Geometry check sheet. Reference: the model listing, model coordinates, mm. Round coordinates to 2 decimals unless told otherwise and drop trailing zeros. Loops run counter-clockwise (first coordinate to the right, second up) from the corner with the lowest first, then second, coordinate; pieces in that order, holes last.
```python
from build123d import *

# Parameters (mm, degrees)
SKETCH_1_R      = 2
SKETCH_1_R_2    = 1.99
EXTRUDE_1_DEPTH = 3


with BuildPart() as part:
    # 草图1 → 凸台-拉伸1 (new body)
    with BuildSketch(Plane.XY):
        with BuildLine():
            Line((-16.651457747, -45.984160086), (-16.651457747, -35.65505653))
            Line((-16.651457747, -35.65505653), (-36.651457747, -35.65505653))
            Line((-36.651457747, -35.65505653), (-36.651457747, -75.65505653))
            Line((-36.651457747, -75.65505653), (14.818542253, -75.65505653))
            Line((14.818542253, -75.65505653), (39.818542253, -32.353786341))
            Line((39.818542253, -32.353786341), (22.498034177, -22.353786341))
            ThreePointArc((22.498034177, -22.353786341), (8.713172451, -39.144030649), (-9.741633911, -50.605044516))
            ThreePointArc((-9.741633911, -50.605044516), (-14.430925396, -50.140427593), (-16.651457747, -45.984160086))
        make_face()
        with Locations((-26.651457747, -40.65505653)):
            Circle(SKETCH_1_R, mode=Mode.SUBTRACT)
        with Locations((-26.651457747, -50.65505653)):
            Circle(SKETCH_1_R_2, mode=Mode.SUBTRACT)
        with Locations((-20.181457747, -65.65505653)):
            Circle(SKETCH_1_R, mode=Mode.SUBTRACT)
        with Locations((-5.181457747, -65.65505653)):
            Circle(SKETCH_1_R, mode=Mode.SUBTRACT)
        with Locations((16.158288215, -53.334548455)):
            Circle(SKETCH_1_R, mode=Mode.SUBTRACT)
        with Locations((23.658288215, -40.344167398)):
            Circle(SKETCH_1_R, mode=Mode.SUBTRACT)
    extrude(amount=EXTRUDE_1_DEPTH)


solid = part.part
```
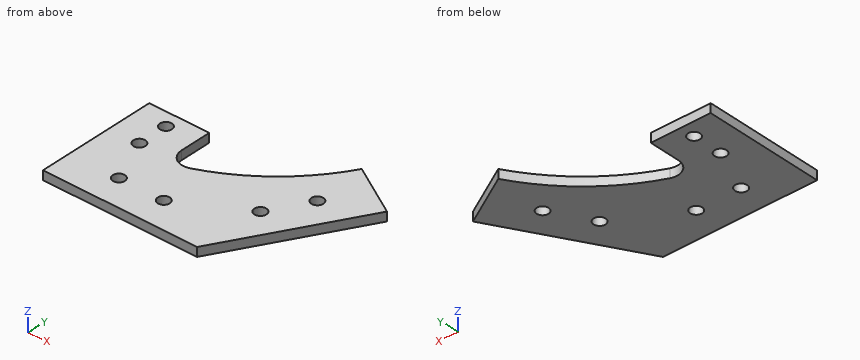
1) Scan lines: line 1 along X through (y, z) = (-41, 0.3); line 2 along Y through (x, z) = (-27.5, 1.05); line 3 along X through (y, z) = (-55, 0.25). Record each from-to range of solid material in increasing order.
Report:
line 1: x = -36.65 to -28.62, -24.68 to -16.65, 6.5 to 21.77, 25.55 to 34.83
line 2: y = -75.66 to -52.46, -48.86 to -42.47, -38.84 to -35.66
line 3: x = -36.65 to 15.05, 17.27 to 26.74
2) Sectioned sample at B-B, the plane y = -47. Record the cut outline in (x, z), then the cut area to 3 significant figures.
Report:
outline: (-36.65, 0) - (-16.55, 0) - (-16.55, 3) - (-36.65, 3) - close; (-2.35, 0) - (31.36, 0) - (31.36, 3) - (-2.35, 3) - close
area: 161 mm2
3) Sectioned sample at C-C, the plane x = -10.5. Record the cut outline in (y, z), then the cut area to 3 significant figures.
Report:
outline: (-75.66, 0) - (-50.85, 0) - (-50.85, 3) - (-75.66, 3) - close
area: 74.4 mm2
4) Sectioned sample at D-D, the plane y = -37. Record the cut outline in (x, z).
Report:
outline: (-36.65, 0) - (-16.65, 0) - (-16.65, 3) - (-36.65, 3) - close; (11.05, 0) - (37.14, 0) - (37.14, 3) - (11.05, 3) - close
5) Gauge pin test, flat ends, axial feed: pin 1 (1 mm diameter, centred on x = 18.5, z = 1, fed in from +Y); pin 2 (5 mm diameter, centred on x = -5.18, y = -65.66, fed in from -Z); pin 3 (3 mm diameter, centred on x = -26.65, y = -50.66, fed in from -Z). Record the tip position at first contact, or that the pin passes through.
Report:
pin 1: stops at y = -27.79
pin 2: stops at z = 0
pin 3: passes through
6) Sectioned sample at A-A, the plane z = 0.85. Record the cut outline in (x, y).
Report:
outline: (-36.65, -75.66) - (14.82, -75.66) - (39.82, -32.35) - (22.5, -22.35) arc R66.6 cw to (-9.74, -50.61) arc R5 cw to (-16.65, -45.98) - (-16.65, -35.66) - (-36.65, -35.66) - close; hole circle Ø4 at (-26.65, -40.66); hole circle Ø3.98 at (-26.65, -50.66); hole circle Ø4 at (-20.18, -65.66); hole circle Ø4 at (-5.18, -65.66); hole circle Ø4 at (16.16, -53.33); hole circle Ø4 at (23.66, -40.34)
